For this review, take the finished solid that the model builds, in its own axes (mm). A direction names the side the tool comes from. Give positions to 0.01 mm unless a question says otherwise; leave off trailing zeros. Loops run counter-clockwise (first coordinate to the right, second up) from the corner with the lowest first, then second, coordinate; pieces in that order, holes last. Notation, with made-up numbers: (74, 41) - (86, 41) arc R15 ccw to (86, 48) - close; hole circle Ø7 at (27.25, 32.5). An arc over 180 degrees is marked (long way). Answer as CSV lines item,"result".
Autodesk Inventor part; units mm, degrees
ref_plane "to_housing_XY" through (0, 0, 0) normal (1, 0, 0) x (0, 0, -1)
ref_plane "to_housing_YZ" through (0, 0, 0) normal (0, 0, -1) x (0, 1, 0)
ref_plane "to_housing_ZX" through (0, 0, 0) normal (0, 1, 0) x (1, 0, 0)
sketch "Sketch_1" plane through (0, 0, 0) normal (0, 0, 1) x (1, 0, 0)
  line L0 (4.8, 0) -> (0.2, 0)
  arc A0 (0, 4.2) -> (0.2, 4) centre (0.2, 4.2) ccw
  line L1 (0.2, 4) -> (4.8, 4)
  arc A1 (4.8, 4) -> (5, 4.2) centre (4.8, 4.2) ccw
  line L2 (5, 4.2) -> (5, 5.28)
  line L3 (5, 5.28) -> (4.84, 5.28)
  line L4 (4.84, 5.28) -> (4.84, 7.056)
  line L5 (4.84, 7.056) -> (5, 7.056)
  line L6 (5, 7.056) -> (5, 7.8)
  arc A2 (5, 7.8) -> (4.8, 8) centre (4.8, 7.8) ccw
  line L7 (4.8, 8) -> (0.2, 8)
  arc A3 (0.2, 8) -> (0, 7.8) centre (0.2, 7.8) ccw
  line L8 (0, 7.8) -> (0, 7.056)
  line L9 (0, 7.056) -> (0.16, 7.056)
  line L10 (0.16, 7.056) -> (0.16, 5.28)
  line L11 (0.16, 5.28) -> (0, 5.28)
  line L12 (0, 5.28) -> (0, 4.2)
revolve "Revolution1" add sketch "Sketch_1" angle 360 about axis through (4.8, 0, 0) along (1, 0, 0)
ref_plane "to_housing_XY" through (0, 0, 0) normal (1, 0, 0) x (0, 0, -1)
ref_plane "to_housing_YZ" through (0, 0, 0) normal (0, 0, -1) x (0, 1, 0)
ref_plane "to_housing_ZX" through (0, 0, 0) normal (0, 1, 0) x (1, 0, 0)
ref_plane "to_housing_center_XY" through (2.5, 0, 0) normal (1, 0, 0) x (0, 0, -1)
ref_plane "to_housing_center_YZ" through (2.5, 0, 0) normal (0, 0, -1) x (0, 1, 0)
ref_plane "to_housing_center_ZX" through (2.5, 0, 0) normal (0, 1, 0) x (1, 0, 0)
properties part number "B688ZZ" material "鋼、合金"
1) Machinability: for faces 1 (the flat face through (0.16, 3, -5)), 2 (the cylindrical face through (2.532, -0.867, -3.905)), which of the approach directions +Z, -Z, +X, -X, +Y, -Y give a long, thin tool a straight path to every point of the face, cutting with its end or side? Answer none if there is none.
From the geometry:
face 1,"-X"
face 2,"+X, -X"
2) Wall thickness on line 1 (Z direction, x = 4.9, y = 0); line 2 (X direction, y = -0.5, z = 5.75); line 3 (Z direction, x = 0.9, y = -3): over which ranges is each line inside the solid? List them lowest first. Write a range as from..to.
From the geometry:
line 1,"z = -7.97..-7.06, -5.28..-4.03, 4.03..5.28, 7.06..7.97"
line 2,"x = 0.16..4.84"
line 3,"z = -7.42..-2.65, 2.65..7.42"
3) Draft analysis for pull direction Y (two halves, no side actions). For faces 3 (the flat face through (0, -6, -4)), 4 (the flat face through (4.84, 3, -5)), 5 (the cylindrical face through (2.47, -1.73, 7.81)), state which applies: pulls with the +Y half, pulls with the -Y half, needs draft (parallel to the pull), parting line crosses it, or undercut.
From the geometry:
face 3,"needs draft"
face 4,"undercut"
face 5,"parting line crosses it"
4) Insertion check: P1, Ø1, axis at x = 2, z = -6, coming from the -Y side; P2, Ø4, axis at y = -0.5, z = 2.5, coming from the -X side; P3, Ø3, axis at x = 3, z = -3, coming from the -Y side; P4, Ø6.5, axis at y = 0, z = 0, coming from the -X side. Each pin has a flat end and moves straight along its axis. Give the tip position at first contact, or say it passes through.
From the geometry:
P1,"stops at y = -5.81"
P2,"stops at x = 0"
P3,"stops at y = -7.86"
P4,"passes through"
5) Consider section C-C on x = 1.15. Write out the cut boundary in (y, z), and give its area (3 significant figures).
From the geometry:
outline,"circle Ø16 at (0, 0); hole circle Ø8 at (0, 0)"
area,"151 mm^2"
